Can you work these out from the model? Positions are in its coordinate system, mm. Face numbers are marked on the shaded views. A direction names the side the tool comes from. Round coordinates to 2 decimals unless told otherwise and drop trailing zeros. Order: outer loops, then holes, each group sorted by start corner. A loop starts at its lowest first (then second) coordinate and runs counter-clockwise, first axis right, second up. Notation, with made-up numbers: (-5, 64) -> (40, 64) arc R15 cw to (40, 77) -> close; hole circle Ø5 at (-28.5, 39). An arc over 180 degrees is marked (long way). One line per item, written item: value.
Autodesk Inventor part; units mm, degrees
ref_plane "Work Plane1" through (0, 304.8, 0) normal (0, 1, 0) x (-1, 0, 0)
ref_plane "Work Plane2" through (0, 0, -213.36) normal (0, 0, 1) x (1, 0, 0)
ref_plane "YZ Plane" through (0, 0, 0) normal (1, 0, 0) x (0, 1, 0)
sketch "Sketch1" plane through (0, 0, 0) normal (0, 1, 0) x (-1, 0, 0)
  line L0 (381, -209.55) -> (-381, -209.55)
  line L1 (-381, -209.55) -> (-381, 247.65)
  line L2 (-381, 247.65) -> (381, 247.65)
  line L3 (381, 247.65) -> (381, -209.55)
  point P0 (0, 0)
  dimension "d0" = 762
extrude "Extrusion1" add sketch "Sketch1" along normal blind 304.8
ref_plane "Work Plane1" through (0, 304.8, 0) normal (0, 1, 0) x (-1, 0, 0)
sketch "Sketch2" plane through (0, 304.8, 0) normal (0, 1, 0) x (-1, 0, 0)
  line L0 (-254, -51.5336) -> (-330.2, -51.5336)
  line L1 (-330.2, -51.5336) -> (-330.2, -178.5336)
  line L2 (-330.2, -178.5336) -> (-254, -178.5336)
  line L3 (-254, -178.5336) -> (-254, -51.5336)
  line L4 (-381, 247.65) -> (-381, -209.55)
  line L5 (381, 247.65) -> (-381, 247.65)
  point P0 (0, 0)
  dimension "d6" = 127
  dimension "d7" = 76.2
extrude "Extrusion2" cut sketch "Sketch2" against normal blind 304.8
ref_plane "Work Plane2" through (0, 0, -213.36) normal (0, 0, 1) x (1, 0, 0)
sketch "Sketch3" plane through (0, 0, -213.36) normal (0, 0, 1) x (1, 0, 0)
  point P0 (0, 0)
sketch "Sketch4" plane through (0, 0, -213.36) normal (0, 0, 1) x (1, 0, 0)
  line L0 (-123.0782, 274.0785) -> (124.5718, 274.0785) construction
  line L1 (124.5718, 274.0785) -> (124.5718, 26.4285) construction
  line L2 (124.5718, 26.4285) -> (-123.0782, 26.4285) construction
  line L3 (-123.0782, 26.4285) -> (-123.0782, 274.0785) construction
  point P0 (0, 0)
properties part number "Box"
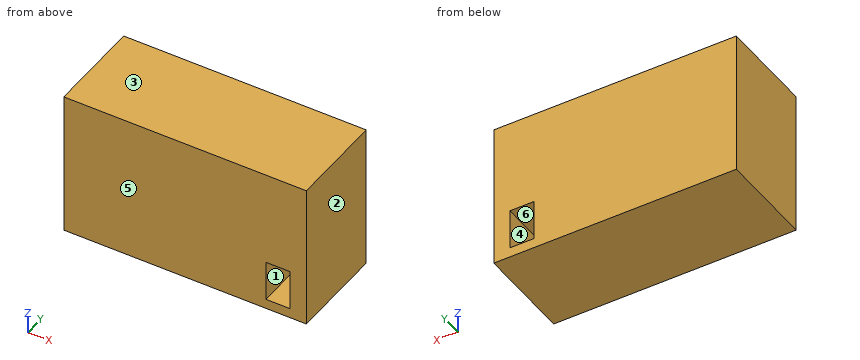
Q1. On a 3-axis mill with a long thin cutter (end or side, diameter ignored), from which of +Z, -Z, +X, -X, +Y, -Y can I reach the whole of each face in a straight line? I mean the marked faces 5 and 6. Say none if no direction works.
Answers below:
face 5: +Z, -Z, +X, -X, -Y
face 6: +Y, -Y
Q2. I want a section at A-A on y = 125. List the corners of the cut face in (x, z) for me, plus the area to 3 significant figures.
Answers below:
outline: (-381, -209.55) -> (381, -209.55) -> (381, 247.65) -> (-381, 247.65) -> close; hole (254, -178.53) -> (330.2, -178.53) -> (330.2, -51.53) -> (254, -51.53) -> close
area: 339,000 mm^2
Q3. I want a section at C-C on x = 291. List the corners of the cut face in (y, z) for me.
Answers below:
outline: (0, -209.55) -> (304.8, -209.55) -> (304.8, -178.53) -> (0, -178.53) -> close; (0, -51.53) -> (304.8, -51.53) -> (304.8, 247.65) -> (0, 247.65) -> close
Q4. I want a section at B-B on z = -63. List the corners of the cut face in (x, y) for me.
Answers below:
outline: (-381, 0) -> (254, 0) -> (254, 304.8) -> (-381, 304.8) -> close; (330.2, 0) -> (381, 0) -> (381, 304.8) -> (330.2, 304.8) -> close
Q5. We'd pull the mould along X, two halves only. Please class the marked faces 1, 2, 3 and 4: released by +X, released by -X, zero draft, split by the parting line, or undercut.
Answers below:
face 1: undercut
face 2: released by +X
face 3: zero draft
face 4: undercut
Q6. Please list where these lines run through material, in increasing order: line 1 along Z through (x, y) = (327, 217); line 2 along X through (y, z) = (216, -118).
Answers below:
line 1: -209.55 to -178.53, -51.53 to 247.65
line 2: -381 to 254, 330.2 to 381
Q7. Will this pin go through, and if not, where does the flat tip stop? pin 1 Ø10 at (x, z) = (-5, -129) entering from -Y.
Answers below:
pin 1: y = 0
